Autodesk Inventor part; units mm, degrees
ref_plane "YZ Plane" through (0, 0, 0) normal (1, 0, 0) x (0, 1, 0)
ref_plane "XZ Plane" through (0, 0, 0) normal (0, 1, 0) x (-1, 0, 0)
ref_plane "XY Plane" through (0, 0, 0) normal (0, 0, 1) x (1, 0, 0)
sketch "Sketch1" plane through (0, 0, 0) normal (0, 0, 1) x (1, 0, 0)
  circle A0 centre (0, 0) radius 15
  dimension "d0" = 30
extrude "Extrusion1" add sketch "Sketch1" along normal blind 1
sketch "Sketch2" plane through (0, 0, 1) normal (0, 0, 1) x (1, 0, 0)
  circle A0 centre (0, 0) radius 12.5
  dimension "d3" = 25
extrude "Extrusion2" add sketch "Sketch2" along normal blind 2
sketch "Sketch3" plane through (0, 0, 3) normal (0, 0, 1) x (1, 0, 0)
  circle A0 centre (0, 0) radius 14.8245
extrude "Extrusion3" add sketch "Sketch3" along normal blind 1
sketch "Sketch4" plane through (0, 0, 4) normal (0, 0, 1) x (1, 0, 0)
  circle A0 centre (0, 0) radius 1.5
  dimension "d8" = 3
extrude "Extrusion4" cut sketch "Sketch4" against normal blind 5
properties part number "Pully Top"
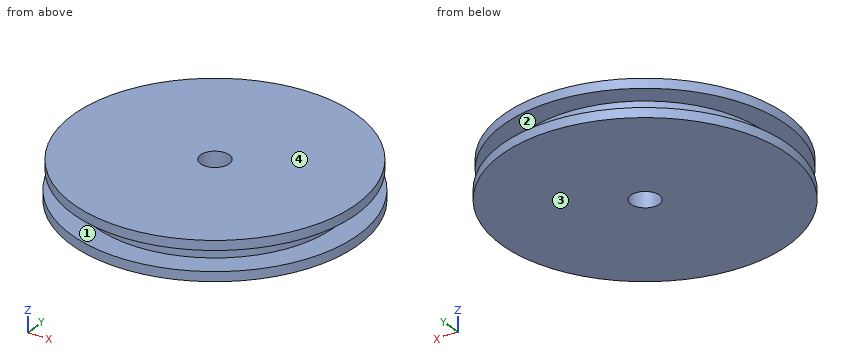
The model under review builds one solid part; all positions refer to its coordinate system, in mm. Face numbers are marked on the shaded views. Coordinates: 2 decimals unless noted, no trailing zeros. Write each loop counter-clockwise with the first axis right and the second up, starting at its lowest first coordinate (ties: lowest second). Pieces come first, ordered by that corner, then holes. Notation, with made-up numbers: (-33, 54) - (25, 54) arc R20 cw to (25, 75) - close; hole circle Ø4 at (82, 5.25). An arc over 180 degrees is marked (long way). Answer in a Markdown table with one row per item. Add a question column.
Q1. To check wall thickness, follow line 1 along Y through (x, z) = (0, 3.05); line 2 along Z through (x, y) = (-11.5, -5.25); line 3 along Y through (x, z) = (0, 2.9). State the ranges of each line that lie inside material, in increasing order. Write a range as from..to.
Q2. Clearance check with flat-ended pins moving along their axes: pin 1 (1 mm diameter, centred on y = -11.5, z = 2, fed in from -X); pin 2 (1.8 mm diameter, centred on x = 0, y = 0, fed in from -Z); pin 3 (1.5 mm diameter, centred on y = -11, z = 2.5, fed in from +X); pin 4 (2 mm diameter, centred on x = -1.5, z = 1, fed in from +Y). State where each tip first meets the part, or that it passes through.
Q3. Draft analysis for pull direction Z (two halves, no side actions). For the marked faces 1, 2, 3 and 4, state which applies: +Z half, -Z half, draft (parallel to the pull), parting line (faces both ways), or undercut.
Q4. Consider section D-D on x = -4.25. Give the boundary of the cut face in (y, z), then the cut area to 3 significant figures.
Q5. Consider section A-A on x = 0. Give the boundary of the cut face in (y, z).
Q6. Consider section C-C on z = 2. Give the boundary of the cut face in (x, y), then the cut area to 3 significant figures.
Answers below:
| question | item | result |
|---|---|---|
| 1 | line 1 | -14.82..-1.5, 1.5..14.82 |
| 1 | line 2 | 0..1, 3..4 |
| 1 | line 3 | -12.5..-1.5, 1.5..12.5 |
| 2 | pin 1 | x = -5.94 |
| 2 | pin 2 | through |
| 2 | pin 3 | x = 10.52 |
| 2 | pin 4 | y = 14.99 |
| 3 | face 1 | undercut |
| 3 | face 2 | undercut |
| 3 | face 3 | -Z half |
| 3 | face 4 | +Z half |
| 4 | outline | (-14.39, 0) - (14.39, 0) - (14.39, 1) - (11.76, 1) - (11.76, 3) - (14.2, 3) - (14.2, 4) - (-14.2, 4) - (-14.2, 3) - (-11.76, 3) - (-11.76, 1) - (-14.39, 1) - close |
| 4 | area | 104 mm² |
| 5 | outline | (-15, 0) - (-1.5, 0) - (-1.5, 4) - (-14.82, 4) - (-14.82, 3) - (-12.5, 3) - (-12.5, 1) - (-15, 1) - close; (1.5, 0) - (15, 0) - (15, 1) - (12.5, 1) - (12.5, 3) - (14.82, 3) - (14.82, 4) - (1.5, 4) - close |
| 6 | outline | circle Ø25 at (0, 0); hole circle Ø3 at (0, 0) |
| 6 | area | 484 mm² |
